Job drawing, mm, ordinate dimensions from the low corner. One solid piece. A direction names the side the tool comes from. Give positions to 0.01 mm unless a question says otherwise; leave off trailing zeros. Loops run counter-clockwise (first coordinate to the right, second up) from the corner with the lowest first, then second, coordinate; pieces in that order, holes last. Notation, with made-up numbers: (37, -10) -> (49, -10) arc R30 ccw to (49, 15) -> close; hole circle Ø1 at (41, 51.5). An arc over 180 degrees is marked (long way). Answer as a JSON object with one key per item and string values. Group by question number.
Q1. Band-saw the part on B-B, the plane x = 25. Write the cut outline in (y, z).
Q2. Drop flat-ended pins along their axis: pin 1 (1.5 mm diameter, centred on x = 5.5, z = 3, fed in from +Y) (1 decimal); pin 2 (5 mm diameter, centred on x = 7.68, y = 15, fed in from +Z); pin 3 (8 mm diameter, centred on x = 41.5, y = 25.5, fed in from -Z); pin 4 (1 mm diameter, centred on y = 12.5, z = 2.5, fed in from -X). Give the stop position or say it passes through.
Q3. Band-saw the part on A-A, the plane y = 25. Write the cut outline in (x, z), plus the area to 3 significant figures.
Q4. Wall check: probe 1 along Y at (x, z) = (27, 6.75) (1 decimal); probe 2 along X at (y, z) = (13, 7.75) (1 decimal); probe 3 along Y at (x, z) = (7.5, 7.75) (1 decimal). Give the ranges that are in metal, low to high. Write a range as from..to.
Q5. Band-saw the part on D-D, the plane x = 9.5. Write the cut outline in (y, z) (1 decimal).
Q6. Tool access for the marked faces 1 and 2: list every direction of +Z, -Z, +X, -X, +Y, -Y with a clear straight run to the whole face (end or side of a thin tool).
Q7. Band-saw the part on C-C, the plane z = 6.25. Write the cut outline in (x, y), plus the area to 3 significant figures.
Q8. Two-plate mould, pull along X, no slides. Class the marked faces 3, 4 and 5: pulls with the +X half, pulls with the -X half, needs draft (parallel to the pull), parting line crosses it, or undercut.
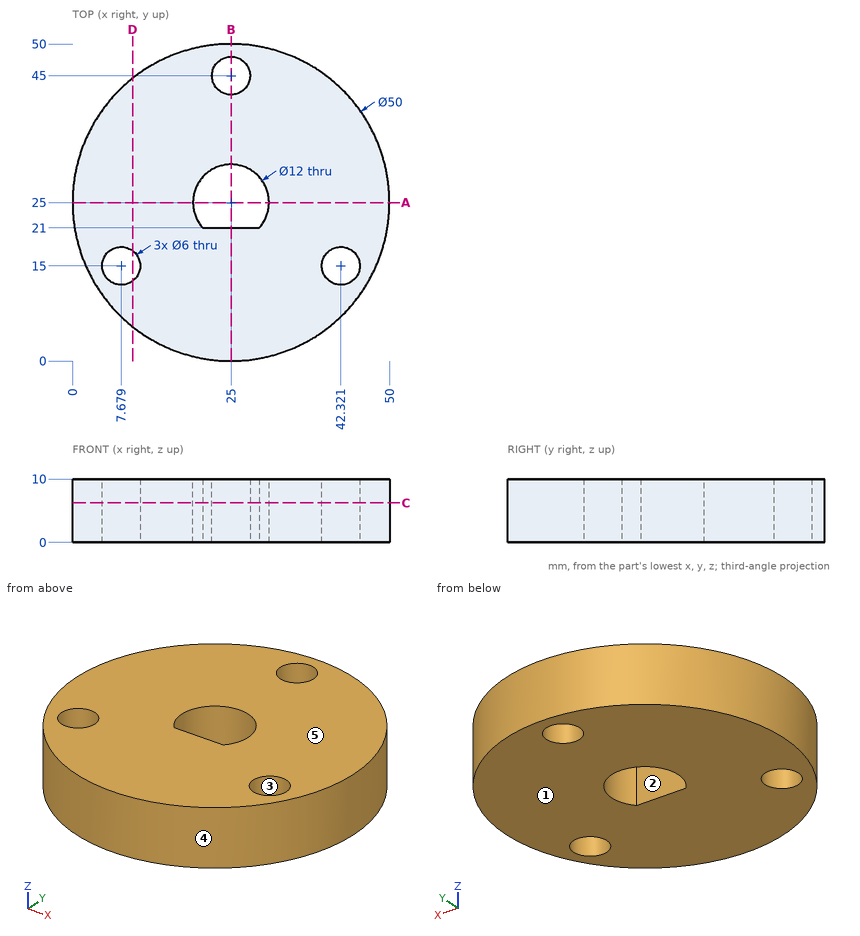
Worked answers:
{
 "1": {"outline": "(0, 0) -> (21, 0) -> (21, 10) -> (0, 10) -> close; (31, 0) -> (42, 0) -> (42, 10) -> (31, 10) -> close; (48, 0) -> (50, 0) -> (50, 10) -> (48, 10) -> close"},
 "2": {"pin 1": "y = 41.5", "pin 2": "through", "pin 3": "z = 0", "pin 4": "x = 3.07"},
 "3": {"outline": "(0, 0) -> (19, 0) -> (19, 10) -> (0, 10) -> close; (31, 0) -> (50, 0) -> (50, 10) -> (31, 10) -> close", "area": "380 mm2"},
 "4": {"probe 1": "0.1..21, 30.7..42.8, 47.2..49.9", "probe 2": "3.1..5.4, 9.9..40.1, 44.6..46.9", "probe 3": "7.1..12, 18..42.9"},
 "5": {"outline": "(5.4, 0) -> (12.6, 0) -> (12.6, 10) -> (5.4, 10) -> close; (17.4, 0) -> (44.6, 0) -> (44.6, 10) -> (17.4, 10) -> close"},
 "6": {"face 1": "-Z, +X, -X, +Y, -Y", "face 2": "+Z, -Z"},
 "7": {"outline": "circle Ø50 at (25, 25); hole circle Ø6 at (7.68, 15); hole (20.53, 21) -> (29.47, 21) arc R6 ccw (long way) to start; hole circle Ø6 at (25, 45); hole circle Ø6 at (42.32, 15)", "area": "1,780 mm2"},
 "8": {"face 3": "undercut", "face 4": "parting line crosses it", "face 5": "needs draft"}
}
